Model file for the job. Use its own axes, mm. Give positions to 0.01 mm unless a question says otherwise; leave off trailing zeros. Loops run counter-clockwise (first coordinate to the right, second up) from the corner with the lowest first, then second, coordinate; pieces in that order, holes last. Notation, with made-up numbers: (-28.5, -30.75) - (25.5, -30.75) arc R36 ccw to (25.5, 3.25) - close; hole circle Ø2 at (64.5, 53). An arc over 180 degrees is marked (long way). Use a Markdown table: item, result.
from build123d import *

# Parameters (mm, degrees)
F0_R      = 33
F1_DEPTH  = 9
F2_SIZE   = 2.2
F1_FACE_R = 33
F3_DEPTH  = 25


with BuildPart() as f1:
    # F0 (on Right) → F1 (new body)
    with BuildSketch(Plane.YZ):
        Circle(F0_R)
    extrude(amount=F1_DEPTH)

    # F2
    f2_edges = [f1.edges().sort_by_distance(p)[0] for p in [
        (9, -33, 0),
    ]]
    chamfer(f2_edges, length=F2_SIZE)

    # F1_face (on face) → F3 (join)
    with BuildSketch(Plane(origin=(0, 0, 0), x_dir=(0, 1, 0), z_dir=(-1, 0, 0))):
        Circle(F1_FACE_R)
    extrude(amount=F3_DEPTH)


solid = f1.part
(1) Pin check, flat tips, straight feed: P1, Ø2, axis at y = 24.5, z = -26, coming from the -X side; P2, Ø1, axis at x = -9, y = 21.5, coming from the -Z side; P3, Ø5, axis at x = -16.5, y = 15, coming from the -Z side; P4, Ø2, axis at x = 3.5, z = 14.5, coming from the +Y side. Stop position of each tip, or through.
Computed:
| item | result |
|---|---|
| P1 | through |
| P2 | z = -25.46 |
| P3 | z = -30.54 |
| P4 | y = 30.11 |
(2) Drill centre lines: probe 1 along Y at (x, z) = (-3, -1); probe 2 along Z at (x, y) = (5, 26). Where is each one in solid material? Low to high. Write a range as [from, to].
Computed:
| item | result |
|---|---|
| probe 1 | [-32.98, 32.98] |
| probe 2 | [-20.32, 20.32] |
(3) Slice it at A-A, the plane x = -7. Write the cut outline in (y, z).
Computed:
| item | result |
|---|---|
| outline | circle Ø66 at (0, 0) |
